from build123d import *

# Parameters (mm, degrees)
SKETCH1_R           = 37.5
BOSS_EXTRUDE1_DEPTH = 150
CUT_EXTRUDE1_START  = 150
SKETCH2_R           = 25
CUT_EXTRUDE1_DEPTH  = 145
SKETCH3_R           = 50
BOSS_EXTRUDE2_DEPTH = 3
FILLET1_R           = 10


with BuildPart() as part:
    # Sketch1 → Boss-Extrude1 (new body)
    with BuildSketch(Plane.XY):
        Circle(SKETCH1_R)
    extrude(amount=BOSS_EXTRUDE1_DEPTH)

    # Sketch2 → Cut-Extrude1 (cut)
    with BuildSketch(Plane.XY.offset(CUT_EXTRUDE1_START)):
        Circle(SKETCH2_R)
    extrude(amount=-CUT_EXTRUDE1_DEPTH, mode=Mode.SUBTRACT)

    # Sketch3 → Boss-Extrude2 (add)
    with BuildSketch(Plane.XY):
        Circle(SKETCH3_R)
    extrude(amount=BOSS_EXTRUDE2_DEPTH)

    # Fillet1
    fillet1_edges = [part.edges().sort_by_distance(p)[0] for p in [
        (-37.5, 0, 3),
    ]]
    fillet(fillet1_edges, radius=FILLET1_R)


solid = part.part
Geometry: final body of the model. Coordinates: model frame, mm. A direction names the side the tool comes from. Round coordinates to 2 decimals unless told otherwise and drop trailing zeros. Loops run counter-clockwise (first coordinate to the right, second up) from the corner with the lowest first, then second, coordinate; pieces in that order, holes last. Notation, with made-up numbers: M 10,49.5 L 24,49.5 A21 ccw 24,72.5 Z; hole C -11,-10.75 d3. An arc over 180 degrees is marked long. Put each result on its own line as item: value. Start each with the question number.
(1) Material intervals for line 1 along Y through (x, z) = (0, 100); line 2 along Z through (x, y) = (7, 17); line 3 along Y through (x, z) = (-14, 30.5), sorted ascending. Write a range as [from, to].
(2) Section query A-A (x = 0). Return loops of the section in (y, z).
(3) Contact query for flat-ended pins moving along their axis: pin 1 Ø8 at (x, y) = (-9.5, -7) entering from +Z; pin 2 Ø2 at (x, z) = (-18.5, 45) entering from +Y; pin 3 Ø12 at (x, z) = (-5.5, 30) entering from -Y. Output: stop coordinate, or through.
(4) Set-up query: faces 1 (the face through (44.2, -18.3, 3)), 2 (the face through (47.69, 15.02, 1.48)). Return all of +Z, -Z, +X, -X, +Y, -Y with unobstructed straight access to the full face (end or side cutting, diameter ignored); none if empty.
(5) Section query C-C (z = 127.5). Return loops of the section in (x, y).
(6) Draft query along X for faces 3 (the face through (23.846, 7.509, 78.515)), 4 (the face through (-4.88, 37.18, 80.54)), 5 (the face through (24, -8, 150)). Return one class per face: +X half, -X half, draft (parallel to the pull), parting line (faces both ways), or undercut.
Findings below:
1. line 1: y = [-37.5, -25], [25, 37.5]
1. line 2: z = [0, 5]
1. line 3: y = [-34.79, -20.71], [20.71, 34.79]
2. outline: M -50,0 L 50,0 L 50,3 L 47.5,3 A10 cw 37.5,13 L 37.5,150 L 25,150 L 25,5 L -25,5 L -25,150 L -37.5,150 L -37.5,13 A10 cw -47.5,3 L -50,3 Z
3. pin 1: stops at z = 5
3. pin 2: stops at y = 33.17
3. pin 3: stops at y = -37.5
4. face 1: +Z
4. face 2: +Z, -Z
5. outline: C 0,0 d75; hole C 0,0 d50
6. face 3: undercut
6. face 4: parting line
6. face 5: draft
